For this review, take the finished solid that the model builds, in its own axes (mm). Round coordinates to 2 decimals unless told otherwise and drop trailing zeros. Write each loop counter-clockwise with the first axis right and the second up, starting at its lowest first coordinate (ties: lowest second). Pieces come first, ordered by that corner, then holes. Notation, with made-up numbers: (34.5, 79) -> (72.5, 79) arc R22 cw to (72.5, 102) -> close; hole circle Ø1 at (76, 65). An arc over 180 degrees is marked (long way). Answer as CSV lines item,"result". Start each with the question number.
Item 1: Wall thickness on probe 1 along Z at (x, y) = (-128.5, 1.7); probe 2 along X at (y, z) = (2.1, -114.5); probe 3 along Z at (x, y) = (-76, 2.75): over which ranges is each line inside the solid? List them lowest first. Write a range as from..to.
Item 2: Take a section at C-C on y = 2.55. Count the separate pieces of the cut face and the enclosed holes in it, then the cut area to 3 significant figures.
Item 3: Take a section at A-A on z = -110.5. Give the boundary of the cut face in (x, y) (3 decimals), then the cut area to 3 significant figures.
Item 4: For pin 1 Ø1.8 at (x, z) = (-117.38, -130.54) entering from +Y, flat-tipped, find the tip position at first contact; note if it passes through.
Item 5: Take a section at B-B on x = -100. Give the boundary of the cut face in (y, z) (3 decimals).
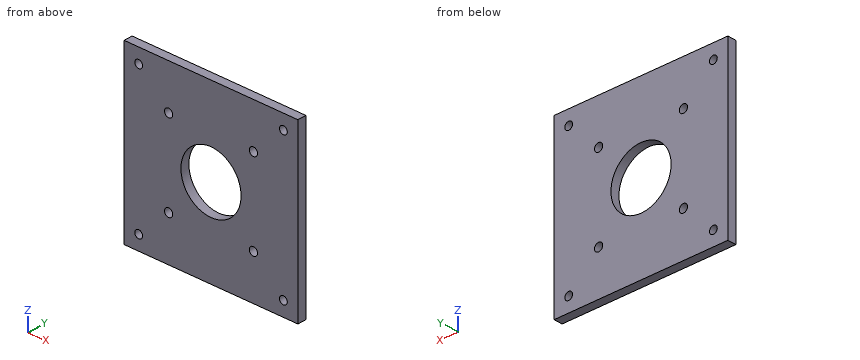
Autodesk Inventor part; units mm, degrees
ref_plane "YZ Plane" through (0, 0, 0) normal (1, 0, 0) x (0, 1, 0)
ref_plane "XZ Plane" through (0, 0, 0) normal (0, 1, 0) x (-1, 0, 0)
ref_plane "XY Plane" through (0, 0, 0) normal (0, 0, 1) x (1, 0, 0)
sketch "Sketch1" plane through (0, 0, 0) normal (0, 1, 0) x (-1, 0, 0)
  circle A0 centre (86.3758, -99.5417) radius 1.5
  circle A1 centre (117.3758, -99.5417) radius 1.5
  circle A2 centre (117.3758, -130.5417) radius 1.5
  circle A3 centre (86.3758, -130.5417) radius 1.5
  circle A4 centre (101.8758, -115.0417) radius 11
  line L0 (133.6258, -146.7917) -> (70.1258, -146.7917)
  line L1 (70.1258, -146.7917) -> (70.1258, -83.2917)
  line L2 (70.1258, -83.2917) -> (133.6258, -83.2917)
  line L3 (133.6258, -83.2917) -> (133.6258, -146.7917)
  line L4 (80.7258, -93.8917) -> (123.0258, -93.8917) construction
  line L5 (123.0258, -93.8917) -> (123.0258, -136.1917) construction
  line L6 (123.0258, -136.1917) -> (80.7258, -136.1917) construction
  line L7 (80.7258, -136.1917) -> (80.7258, -93.8917) construction
  line L8 (80.7258, -136.1917) -> (123.0258, -93.8917) construction
  line L9 (123.0258, -136.1917) -> (80.7258, -93.8917) construction
  circle A5 centre (75.4258, -88.5917) radius 1.4224
  circle A6 centre (75.4258, -141.4917) radius 1.4224
  circle A7 centre (128.3258, -141.4917) radius 1.4224
  circle A8 centre (128.3258, -88.5917) radius 1.4224
  point P0 (0, 0)
  dimension "d9" = 63.5
  dimension "d11" = 2.8448
  dimension "d12" = 2.8448
  dimension "d19" = 63.5
  dimension "d20" = 2.8448
  dimension "d21" = 2.8448
extrude "Extrusion1" add sketch "Sketch1" along normal blind 3.175
ref_plane "Work Plane1" through (-70.1258, 0, -115.0417) normal (0, 0, -1) x (-1, 0, 0)
Output values:
1,probe 1,"z = -146.79..-142.9, -140.08..-90, -87.18..-83.29"
1,probe 2,"x = -133.63..-112.86, -90.89..-70.13"
1,probe 3,"z = -146.79..-142.79, -140.19..-89.89, -87.29..-83.29"
2,separate pieces,"1"
2,enclosed holes,"9"
2,area,"3,600 mm^2"
3,outline,"(-133.626, 0) -> (-111.894, 0) -> (-111.894, 3.175) -> (-133.626, 3.175) -> close; (-91.857, 0) -> (-70.126, 0) -> (-70.126, 3.175) -> (-91.857, 3.175) -> close"
3,area,"138 mm^2"
4,pin 1,"passes through"
5,outline,"(0, -146.792) -> (3.175, -146.792) -> (3.175, -125.881) -> (0, -125.881) -> close; (0, -104.203) -> (3.175, -104.203) -> (3.175, -83.292) -> (0, -83.292) -> close"
